Autodesk Inventor part; units mm, degrees
ref_plane "YZ Plane" through (0, 0, 0) normal (1, 0, 0) x (0, 1, 0)
ref_plane "XZ Plane" through (0, 0, 0) normal (0, 1, 0) x (-1, 0, 0)
ref_plane "XY Plane" through (0, 0, 0) normal (0, 0, 1) x (1, 0, 0)
sketch "Skizze1" plane through (0, 0, 0) normal (1, 0, 0) x (0, 1, 0)
  circle A0 centre (0, 0) radius 12.15
  line L0 (0, 16.95) -> (23.4061, 16.95) construction
  line L1 (0, 20.45) -> (9, 20.45)
  arc A1 (16, 0) -> (9, 13.2288) centre (0, 0) ccw
  line L2 (9, 13.2288) -> (9, 20.45)
  line L3 (0, 20.45) -> (0, 12.15)
  line L4 (0, 28.63) -> (0, -28.63)
  line L5 (0, 0) -> (16, 0)
  line L6 (0, -20.45) -> (9, -20.45)
  arc A2 (9, -13.2288) -> (16, 0) centre (0, 0) ccw
  line L7 (9, -13.2288) -> (9, -20.45)
  line L8 (0, -20.45) -> (0, -12.15)
  point P0 (0, -12.15)
  dimension "d0" = 24.3
  dimension "d1" = 16.95
  dimension "d2" = 20.45
  dimension "d3" = 9
  dimension "d4" = 16
extrude "Extrusion1" add sketch "Skizze1" against normal blind 7 contours L5 A2 L7 L6 L4 A0 | A0 L3 L1 L2 A1 L5
sketch "Skizze2" plane through (0, 0, 0) normal (0, 1, 0) x (-1, 0, 0)
  circle A0 centre (3.5, 16.95) radius 1.7
  circle A1 centre (3.5, -16.95) radius 1.7162
  line L0 (0, 20.45) -> (7, 20.45)
  line L1 (-1.4, 0) -> (8.4, 0)
  point P0 (0, 0)
  point P1 (3.5, 20.45)
  point P2 (3.5, 20.45)
  dimension "d9" = 33.9
  dimension "d10" = 3.4
extrude "Extrusion2" cut sketch "Skizze2" along normal through all
sketch "Skizze3" plane through (0, 0, 0) normal (1, 0, 0) x (0, 1, 0)
  arc A0 (9, -13.2288) -> (9, 13.2288) centre (0, 0) ccw
  arc A1 (9, -13.2288) -> (9, 13.2288) centre (0, 0) ccw
  line L0 (17, 9.5) -> (12.8744, 9.5)
  line L1 (12.8744, 9.5) -> (12.8744, -9.5)
  line L2 (12.8744, -9.5) -> (17, -9.5)
  line L3 (17, -9.5) -> (17, 9.5)
  line L4 (0, -12.15) -> (0, -20.45)
  point P0 (12.8744, -9.5)
  dimension "d14" = 19
  dimension "d22" = 17
extrude "Extrusion3" add sketch "Skizze3" against normal up to surface (7 mm away) contours A0 L0 L3 L2
sketch "Skizze4" plane through (0, 17, 9.5) normal (0, 1, 0) x (1, 0, 0)
  circle A0 centre (-3.5, 5) radius 2
  circle A1 centre (-3.5, 14) radius 2
  line L0 (0, 9.5) -> (-10.2525, 9.5)
  line L1 (0, 19) -> (-7, 19)
  point P0 (-3.5, 19)
  dimension "d17" = 4
  dimension "d18" = 9
extrude "Extrusion4" cut sketch "Skizze4" against normal blind 4
properties part number "Motorhalter"
Here's how the part is built. I have some questions about the finished solid (model axes, mm). A direction names the side the tool comes from. Coordinates: 2 decimals unless noted, no trailing zeros. Loops run counter-clockwise (first coordinate to the right, second up) from the corner with the lowest first, then second, coordinate; pieces in that order, holes last.
1. For faces 4 (the flat face through (-4, 13, 4)), 5 (the flat face through (-3, 15, 9.5)), 6 (the flat face through (-3, 15, -9.5)), which set-ups out of +Z, -Z, +X, -X, +Y, -Y let a thin tool reach every point of the face, with its end or its side?
2. Imagine slicing it at C-C, the plane x = -3.5. Please give me the cut outline in (y, z).
3. If we mould it in two halves opening along Z, with no side actions, what happens to faces 1 (the cylindrical face through (-3.451, 11.122, 11.502)), 2 (the cylindrical face through (-5.1, 15, -3.3)), 3 (the flat face through (-7, 14, 0))? For each: pulls with the +Z half, pulls with the -Z half, needs draft (parallel to the pull), parting line crosses it, or undercut.
4. Imagine slicing it at B-B, the plane y = 8.5. Please give me the cut outline in (x, z), and give its area (3 significant figures).
5. For P1, Ø2, axis at x = -4, y = 15.5, coming from the +Z side; P2, Ø4, axis at x = -3.5, z = 16.95, coming from the +Y side; P3, Ø3, axis at x = -3.5, z = -4.5, coming from the +Y side, each with a flat end and sliding along its axis, tell me the tip position at first contact or that it passes through.
6. Imagine slicing it at A-A, the plane z = 16.95. Please give me the cut outline in (x, y), and give its area (3 significant figures).
7. I need wall thicknesses on L1, parallel to Z at x = -3.5, y = 15.3; L2, parallel to Z at x = -3.5, y = 5.5; L3, parallel to Z at x = -5, y = 13.5. Which ranges of each line are inside material? Lowest first, please.
8. Imagine slicing it at D-D, the plane z = -16.95. Please give me the cut outline in (x, y).
Taken from the geometry:
1. face 4: +Y
1. face 5: +Z, +X, -X, +Y
1. face 6: -Z, +X, -X, +Y
2. outline: (0, -20.45) - (9, -20.45) - (9, -18.67) - (0, -18.67) - close; (0, -15.23) - (9, -15.23) - (9, -13.23) arc R16 ccw to (12.87, -9.5) - (17, -9.5) - (17, -6.5) - (13, -6.5) - (13, -2.5) - (17, -2.5) - (17, 2.5) - (13, 2.5) - (13, 6.5) - (17, 6.5) - (17, 9.5) - (12.87, 9.5) arc R16 ccw to (9, 13.23) - (9, 15.25) - (0, 15.25) - (0, 12.15) arc R12.15 cw to (0, -12.15) - close; (0, 18.65) - (9, 18.65) - (9, 20.45) - (0, 20.45) - close
3. face 1: pulls with the +Z half
3. face 2: undercut
3. face 3: needs draft
4. outline: (-7, -20.45) - (0, -20.45) - (0, -8.68) - (-7, -8.68) - close; (-7, 8.68) - (0, 8.68) - (0, 20.45) - (-7, 20.45) - close; hole circle Ø3.43 at (-3.5, -16.95); hole circle Ø3.4 at (-3.5, 16.95)
4. area: 146 mm2
5. P1: stops at z = 9.5
5. P2: stops at y = 9
5. P3: stops at y = 13
6. outline: (-7, 0) - (-5.2, 0) - (-5.2, 9) - (-7, 9) - close; (-1.8, 0) - (0, 0) - (0, 9) - (-1.8, 9) - close
6. area: 32.4 mm2
7. L1: z = -9.5 to -6.5, -2.5 to 2.5, 6.5 to 9.5
7. L2: z = -20.45 to -18.67, -15.23 to -10.83, 10.83 to 15.25, 18.65 to 20.45
7. L3: z = -9.5 to -5.82, -3.18 to 3.18, 5.82 to 9.5
8. outline: (-7, 0) - (-5.22, 0) - (-5.22, 9) - (-7, 9) - close; (-1.78, 0) - (0, 0) - (0, 9) - (-1.78, 9) - close
